The listing builds one solid part. Answer for the finished solid, in the listing's coordinates (mm). A direction names the side the tool comes from. Round coordinates to 2 decimals unless told otherwise and drop trailing zeros. Order: outer loops, then holes, each group sorted by start corner. A loop starts at its lowest first (then second) coordinate and runs counter-clockwise, first axis right, second up. Notation, with made-up numbers: (20.5, -14) - (49.5, -14) arc R14 cw to (49.5, 2) - close; hole circle Ø1 at (-28, 63). An arc over 180 degrees is marked (long way). Write item = value, one per line.
from build123d import *

# Parameters (mm, degrees)
F0_R     = 1.75
F1_DEPTH = 3
F2_W     = 10
F2_H     = 3
F3_DEPTH = 10
F4_R     = 1.75
F5_DEPTH = 44.317625


with BuildPart() as f1:
    # F0 (on Top) → F1 (new body)
    with BuildSketch(Plane.XY):
        with BuildLine():
            Line((-5, 26), (-5, 0))
            Line((-5, 0), (5, 0))
            Line((5, 0), (5, 26))
            ThreePointArc((5, 26), (5.585786, 27.414214), (7, 28))
            Line((7, 28), (13, 28))
            ThreePointArc((13, 28), (13.707107, 28.292893), (14, 29))
            Line((14, 29), (14, 29.2))
            ThreePointArc((14, 29.2), (13.707107, 29.907107), (13, 30.2))
            Line((13, 30.2), (10, 30.2))
            ThreePointArc((10, 30.2), (9.487652, 30.05), (8.975305, 30.2))
            Line((8.975305, 30.2), (6.975305, 30.2))
            ThreePointArc((6.975305, 30.2), (6.175305, 31), (6.975305, 31.8))
            Line((6.975305, 31.8), (8.975305, 31.8))
            ThreePointArc((8.975305, 31.8), (9.487652, 31.95), (10, 31.8))
            Line((10, 31.8), (13, 31.8))
            ThreePointArc((13, 31.8), (13.707107, 32.092893), (14, 32.8))
            Line((14, 32.8), (14, 33))
            ThreePointArc((14, 33), (13.707107, 33.707107), (13, 34))
            Line((13, 34), (7, 34))
            ThreePointArc((7, 34), (5.585786, 34.585786), (5, 36))
            Line((5, 36), (5, 40))
            ThreePointArc((5, 40), (0, 49.316625), (-5, 40))
            Line((-5, 40), (-5, 36))
            ThreePointArc((-5, 36), (-5.585786, 34.585786), (-7, 34))
            Line((-7, 34), (-13, 34))
            ThreePointArc((-13, 34), (-13.707107, 33.707107), (-14, 33))
            Line((-14, 33), (-14, 32.8))
            ThreePointArc((-14, 32.8), (-13.707107, 32.092893), (-13, 31.8))
            Line((-13, 31.8), (-10, 31.8))
            ThreePointArc((-10, 31.8), (-9.487652, 31.95), (-8.975305, 31.8))
            Line((-8.975305, 31.8), (-6.975305, 31.8))
            ThreePointArc((-6.975305, 31.8), (-6.175305, 31), (-6.975305, 30.2))
            Line((-6.975305, 30.2), (-8.975305, 30.2))
            ThreePointArc((-8.975305, 30.2), (-9.487652, 30.05), (-10, 30.2))
            Line((-10, 30.2), (-13, 30.2))
            ThreePointArc((-13, 30.2), (-13.707107, 29.907107), (-14, 29.2))
            Line((-14, 29.2), (-14, 29))
            ThreePointArc((-14, 29), (-13.707107, 28.292893), (-13, 28))
            Line((-13, 28), (-7, 28))
            ThreePointArc((-7, 28), (-5.585786, 27.414214), (-5, 26))
        make_face()
        with Locations((0, 43.316625)):
            Circle(F0_R, mode=Mode.SUBTRACT)
    extrude(amount=F1_DEPTH)

    # F2 (on face) → F3 (join)
    with BuildSketch(Plane.XY.offset(3)):
        with Locations((0, 6.5)):
            Rectangle(F2_W, F2_H)
    extrude(amount=F3_DEPTH)

    # F4 (on face) → F5 (cut, through all)
    with BuildSketch(Plane.XZ.offset(-5)):
        with Locations((0, 8)):
            Circle(F4_R)
    extrude(amount=-F5_DEPTH, mode=Mode.SUBTRACT)


solid = f1.part
Q1. Determine the mould class of faces 4 (the face through (-13.715, 28.301, 1.479)), 5 (the face through (-12, 31.8, 1)), 6 (the face through (8, 31.8, 1)), 7 (the face through (0, 7, 13)) for opening direction Y: released by +Y, released by -Y, zero draft, split by the parting line, or undercut.
Model answer:
face_4 = released by -Y
face_5 = undercut
face_6 = undercut
face_7 = zero draft
Q2. Section B-B on x = 0 is taken. Determine the outline of the cut face in (y, z), then the cut area to 3 significant figures.
Model answer:
outline = (0, 0) - (41.57, 0) - (41.57, 3) - (8, 3) - (8, 6.25) - (5, 6.25) - (5, 3) - (0, 3) - close; (5, 9.75) - (8, 9.75) - (8, 13) - (5, 13) - close; (45.07, 0) - (49.32, 0) - (49.32, 3) - (45.07, 3) - close
area = 157 mm^2
Q3. For faces 1 (the face through (10, 34, 1)), 2 (the face through (0, 5, 10)), 3 (the face through (5, 38, 1)), determine the directions among +Z, -Z, +X, -X, +Y, -Y from which every point of the face is accessible in a straight line to the end or side of a thin tool.
Model answer:
face_1 = +Z, -Z, +X, +Y
face_2 = +Z, +X, -X, -Y
face_3 = +Z, -Z, +X
Q4. Flat-ended cylindrical pins translate along their axes: P1, Ø4, axis at x = -1, y = 15, coming from the +Z side; P2, Ø0.9, axis at y = 38.5, z = 1.5, coming from the -X side; P3, Ø1, axis at x = -2, z = 2.5, coming from the +Y side; P4, Ø6.5, axis at y = 11.5, z = 9.5, coming from the -X side. Find the tip coordinate at first contact, or state that the pin passes through.
Model answer:
P1 = 3
P2 = -5
P3 = 49.13
P4 = through
Q5. Section A-A on x = -8 is taken. Determine the outline of the cut face in (y, z), then the cut area to 3 significant figures.
Model answer:
outline = (28, 0) - (30.2, 0) - (30.2, 3) - (28, 3) - close; (31.8, 0) - (34, 0) - (34, 3) - (31.8, 3) - close
area = 13.2 mm^2
Q6. Section D-D on z = 5 is taken. Determine the outline of the cut face in (x, y), then the cut area to 3 significant figures.
Model answer:
outline = (-5, 5) - (5, 5) - (5, 8) - (-5, 8) - close
area = 30.0 mm^2
Q7. Section C-C on y = 7.5 is taken. Determine the outline of the cut face in (x, z).
Model answer:
outline = (-5, 0) - (5, 0) - (5, 13) - (-5, 13) - close; hole circle Ø3.5 at (0, 8)
Q8. Find the intervals of material crossed by line 1 (Z direction, x = 0, y = 7.05); line 2 (Z direction, x = 1, y = 22); line 3 (X direction, y = 19, z = 1.75), in increasing order. Write a range as from..to.
Model answer:
line_1 = 0..6.25, 9.75..13
line_2 = 0..3
line_3 = -5..5
